CAD build for the part. Positions are in the model's coordinates, mm. A direction names the side the tool comes from. Round coordinates to 2 decimals unless told otherwise and drop trailing zeros. Loops run counter-clockwise (first coordinate to the right, second up) from the corner with the lowest first, then second, coordinate; pieces in that order, holes last. Notation, with made-up numbers: M -3,-37.75 L 41,-37.75 A33 cw 41,-6.75 Z; hole C 15,43 d1. An arc over 180 degrees is marked long. Use one line per item in the form item = value.
from build123d import *

# Parameters (mm, degrees)
F0_R     = 38.1
F0_R_2   = 36.83
F0_R_3   = 26.67
F1_DEPTH = 25.4
F0_R_4   = 3.937
F0_R_5   = 1.905
F0_R_6   = 4.191
F2_DEPTH = 15.24


with BuildPart() as f1:
    # F0 (on Front) → F1 (new body)
    with BuildSketch(Plane.XZ):
        Circle(F0_R)
        Circle(F0_R_2, mode=Mode.SUBTRACT)
        Circle(F0_R_2)
        Circle(F0_R_3, mode=Mode.SUBTRACT)
    extrude(amount=F1_DEPTH)

    # F0 (on Front) → F2 (join)
    with BuildSketch(Plane.XZ):
        Circle(F0_R_3)
        with Locations((-13.007903, -12.854781)):
            Circle(F0_R_4, mode=Mode.SUBTRACT)
        with Locations((0, -18.288)):
            Circle(F0_R_4, mode=Mode.SUBTRACT)
        with Locations((13.007903, -12.854781)):
            Circle(F0_R_4, mode=Mode.SUBTRACT)
        with Locations((0, -7.874)):
            Circle(F0_R_5, mode=Mode.SUBTRACT)
        with Locations((-18.288, 0)):
            Circle(F0_R_4, mode=Mode.SUBTRACT)
        with Locations((-7.874, 0)):
            Circle(F0_R_5, mode=Mode.SUBTRACT)
        with Locations((-13.007903, 12.854781)):
            Circle(F0_R_4, mode=Mode.SUBTRACT)
        Circle(F0_R_6, mode=Mode.SUBTRACT)
        with Locations((7.874, 0)):
            Circle(F0_R_5, mode=Mode.SUBTRACT)
        with Locations((0, 7.874)):
            Circle(F0_R_5, mode=Mode.SUBTRACT)
        with Locations((18.288, 0)):
            Circle(F0_R_4, mode=Mode.SUBTRACT)
        with Locations((0, 18.288)):
            Circle(F0_R_4, mode=Mode.SUBTRACT)
        with Locations((12.854781, 13.007903)):
            Circle(F0_R_4, mode=Mode.SUBTRACT)
    extrude(amount=F2_DEPTH)


solid = f1.part
1. Cut at A-A on z = 0. Write the cut outline in (x, y) (3 decimals), and give its area (3 significant figures).
Completed:
outline = M -38.1,-25.4 L -26.67,-25.4 L -26.67,-15.24 L -22.225,-15.24 L -22.225,0 L -38.1,0 Z; M -14.351,-15.24 L -9.779,-15.24 L -9.779,0 L -14.351,0 Z; M -5.969,-15.24 L -4.191,-15.24 L -4.191,0 L -5.969,0 Z; M 4.191,-15.24 L 5.969,-15.24 L 5.969,0 L 4.191,0 Z; M 9.779,-15.24 L 14.351,-15.24 L 14.351,0 L 9.779,0 Z; M 22.225,-15.24 L 26.67,-15.24 L 26.67,-25.4 L 38.1,-25.4 L 38.1,0 L 22.225,0 Z
area = 910 mm2
2. Drop flat-ended pins along their axis: P1, Ø1.5, axis at x = -15, y = -19.5, coming from the -Z side; P2, Ø4.5, axis at x = 7.874, z = 0, coming from the -Y side; P3, Ø1.5, axis at y = -17, z = 18, coming from the +X side; P4, Ø4.5, axis at x = 0, z = -7.874, coming from the +Y side. Give the stop position or say it passes through.
Completed:
P1 = -35.33
P2 = -15.24
P3 = 33.97
P4 = 0
3. Cut at D-D on y = -9.5. State how many separate pieces and enclosed holes the cut face has, and give its area (3 significant figures).
Completed:
separate_pieces = 1
enclosed_holes = 13
area = 4,070 mm2
4. Pull direction X, two halves, no side cores. Call faces 1 (the face through (8, 0, -8)), 2 (the face through (-30.235, -12.522, -23.183)), 3 (the face through (-9.253, -7.513, -11.672)): +X half, -X half, draft (parallel to the pull), parting line (faces both ways), or undercut.
Completed:
face_1 = draft
face_2 = parting line
face_3 = undercut
5. Cut at B-B on y = -21. Write the cut outline in (x, z), and give its area (3 significant figures).
Completed:
outline = C 0,0 d76.2; hole C 0,0 d53.34
area = 2,330 mm2
6. Cut at C-C on x = 7.5. Write the cut outline in (y, z), and give its area (3 significant figures).
Completed:
outline = M -25.4,-37.35 L 0,-37.35 L 0,-1.87 L -15.24,-1.87 L -15.24,-25.59 L -25.4,-25.59 Z; M -25.4,25.59 L -15.24,25.59 L -15.24,1.87 L 0,1.87 L 0,37.35 L -25.4,37.35 Z
area = 1,320 mm2
7. Probe line 1 along Z through (x, y) = (0, -12) (3 decimals); line 2 along Z through (x, y) = (-12, -2.5); line 3 along X through (y, z) = (-9.75, 10). List the from-to ranges inside material, lowest first. Write a range as from..to.
Completed:
line_1 = -38.1..-22.225, -14.351..-9.779, -5.969..-4.191, 4.191..5.969, 9.779..14.351, 22.225..38.1
line_2 = -36.16..-16.66, -9.05..9.05, 16.66..36.16
line_3 = -36.76..-15.72, -10.3..10.31, 15.39..36.76
8. Tool access for faces 4 (the face through (-0.4, -15.24, -5.6)), 5 (the face through (8, -25.4, 26)): list every direction of +Z, -Z, +X, -X, +Y, -Y with a clear straight run to the whole face (end or side of a thin tool).
Completed:
face_4 = -Y
face_5 = +Z, -Z, +X, -X, -Y
